from build123d import *

# Parameters (mm, degrees)
BOSS_EXTRUDE1_DEPTH = 17.5
SKETCH2_R           = 5
CUT_EXTRUDE1_DEPTH  = 36
SKETCH3_R           = 1.65
CUT_EXTRUDE2_DEPTH  = 27
FILLET1_R           = 0.7
SKETCH8_R           = 8
CUT_EXTRUDE5_DEPTH  = 1


with BuildPart() as part:
    # Sketch1 → Boss-Extrude1 (new body, symmetric)
    with BuildSketch(Plane(origin=(0, 0, 0), x_dir=(0, 0, -1), z_dir=(1, 0, 0))):
        Polygon((-20, 26), (-7, 26), (-7, 25), (7, 25), (7, 26), (20, 26), (20, 18), (18, 16), (18, 5), (9.980120734, 5), (5.980120734, 0), (-5.980120734, 0), (-9.980120734, 5), (-18, 5), (-18, 16), (-20, 18), align=None)
    extrude(amount=BOSS_EXTRUDE1_DEPTH, both=True)

    # Sketch2 → Cut-Extrude1 (cut, through all)
    with BuildSketch(Plane(origin=(17.5, 0, 0), x_dir=(0, 0, -1), z_dir=(1, 0, 0))):
        with Locations((0, 13)):
            Circle(SKETCH2_R)
    extrude(amount=-CUT_EXTRUDE1_DEPTH, mode=Mode.SUBTRACT)

    # Sketch3 → Cut-Extrude2 (cut, through all)
    with BuildSketch(Plane(origin=(0, 26, 0), x_dir=(1, 0, 0), z_dir=(0, 1, 0))):
        with Locations((-10.5, 14)):
            Circle(SKETCH3_R)
        with Locations((10.5, 14)):
            Circle(SKETCH3_R)
        with Locations((10.5, -14)):
            Circle(SKETCH3_R)
        with Locations((-10.5, -14)):
            Circle(SKETCH3_R)
    extrude(amount=-CUT_EXTRUDE2_DEPTH, mode=Mode.SUBTRACT)

    # Fillet1
    fillet1_edges = [part.edges().sort_by_distance(p)[0] for p in [
        (-12.15, 26, -14),
        (8.85, 26, -14),
        (8.85, 26, 14),
        (-12.15, 26, 14),
    ]]
    fillet(fillet1_edges, radius=FILLET1_R)

    # Sketch8 → Cut-Extrude5 (cut)
    with BuildSketch(Plane(origin=(17.5, 0, 0), x_dir=(0, 0, -1), z_dir=(1, 0, 0))):
        with Locations((0, 13)):
            Circle(SKETCH8_R)
    cut_extrude5 = extrude(amount=-CUT_EXTRUDE5_DEPTH, mode=Mode.SUBTRACT)

    # Mirror3: Cut-Extrude5 across plane
    add(cut_extrude5.mirror(Plane(origin=(0, 0, 0), x_dir=(0, 0, 1), z_dir=(1, 0, 0))), mode=Mode.SUBTRACT)


solid = part.part
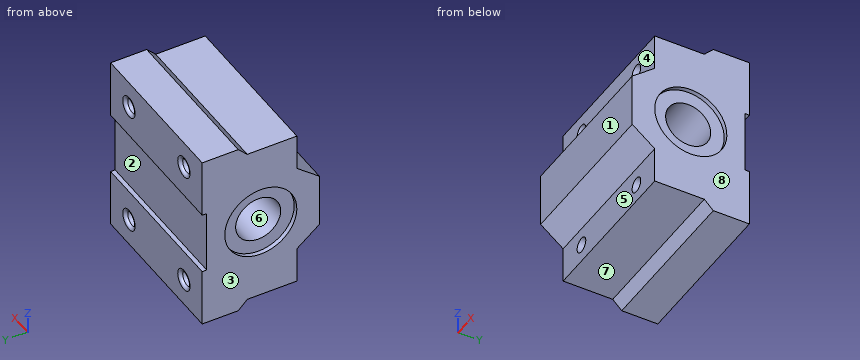
Source: CAD feature listing. Evaluate the final solid. Frame: model axes, mm. Face numbers are marked on the shaded views. A direction names the side the tool comes from. Give positions to 0.01 mm unless a question says otherwise; leave off trailing zeros. Write each loop counter-clockwise with the first axis right and the second up, starting at its lowest first coordinate (ties: lowest second). Pieces come first, ordered by that corner, then holes. Notation, with made-up numbers: M 57.25,59.25 L 76.25,59.25 A22 ccw 76.25,87.25 Z; hole C 56,-38 d1. An arc over 180 degrees is marked long. Answer as a JSON object with one key per item and string values.
Q1. Cut plane A-A, the plane y = 13. Return the cut outline in (x, z).
Geometry check:
{"outline": "M -17.5,-18 L 17.5,-18 L 17.5,-8 L 16.5,-8 L 16.5,-5 L -16.5,-5 L -16.5,-8 L -17.5,-8 Z; M -17.5,8 L -16.5,8 L -16.5,5 L 16.5,5 L 16.5,8 L 17.5,8 L 17.5,18 L -17.5,18 Z; hole C -10.5,-14 d3.3; hole C -10.5,14 d3.3; hole C 10.5,-14 d3.3; hole C 10.5,14 d3.3"}
Q2. Cut plane B-B, the plane x = 10.5. Count the separate pieces of the cut face and the enclosed holes in it, then the cut area to 3 significant figures.
Geometry check:
{"separate pieces": "3", "enclosed holes": "1", "area": "640 mm^2"}
Q3. Cut plane D-D, the plane y = 20.25. Return the cut outline in (x, z), then the cut area to 3 significant figures.
Geometry check:
{"outline": "M -17.5,-20 L 17.5,-20 L 17.5,-3.38 L 16.5,-3.38 L 16.5,3.38 L 17.5,3.38 L 17.5,20 L -17.5,20 L -17.5,3.38 L -16.5,3.38 L -16.5,-3.38 L -17.5,-3.38 Z; hole C -10.5,-14 d3.3; hole C -10.5,14 d3.3; hole C 10.5,-14 d3.3; hole C 10.5,14 d3.3", "area": "1,350 mm^2"}
Q4. Cut plane C-C, the plane z = 14. Return the cut outline in (x, y), then the cut area to 3 significant figures.
Geometry check:
{"outline": "M -17.5,5 L -12.15,5 L -12.15,25.3 A0.7 ccw -12.85,26 L -17.5,26 Z; M -8.85,5 L 8.85,5 L 8.85,25.3 A0.7 ccw 8.15,26 L -8.15,26 A0.7 ccw -8.85,25.3 Z; M 12.15,5 L 17.5,5 L 17.5,26 L 12.85,26 A0.7 ccw 12.15,25.3 Z", "area": "596 mm^2"}
Q5. Mould query, pull axis Z, two halves, no side actions, for the marked faces 6, 7 and 8. Classes: +Z half, -Z half, draft (parallel to the pull), parting line (faces both ways), or undercut.
Geometry check:
{"face 6": "undercut", "face 7": "-Z half", "face 8": "draft"}
Q6. Ray query, line 1 along Z through (x, y) = (-10.5, 18.25); line 2 along Z through (x, y) = (-10.5, 16); line 3 along Y through (x, z) = (-17.1, 0). Return the intervals inside material, ascending.
Geometry check:
{"line 1": "z = -20 to -15.65, -12.35 to 12.35, 15.65 to 20", "line 2": "z = -18 to -15.65, -12.35 to -4, 4 to 12.35, 15.65 to 18", "line 3": "y = 0 to 5, 21 to 25"}
Q7. Access query for the marked faces 1, 2, 3, 4 and 5. Directions: +Z, -Z, +X, -X, +Y, -Y. A direction counts if a zero-diameter tool reaches every point of the face in a straight line with its end or side. Return the directions, or none.
Geometry check:
{"face 1": "+Z, -Z, +X, -X, -Y", "face 2": "+X, -X, +Y", "face 3": "+Z, -Z, -X, +Y, -Y", "face 4": "+Z, +X, -X, -Y", "face 5": "-Z, +X, -X, -Y"}
Q8. Contact query for flat-ended pins moving along their axis: P1, Ø2.5, axis at x = 1, z = -15, coming from the -Y side; P2, Ø3, axis at x = -3.5, y = 9, coming from the +Z side; P3, Ø1.5, axis at x = 7, y = 3.5, coming from the -Z side; P4, Ø8, axis at y = 13, z = 0, coming from the +X side. Output: stop coordinate, or through.
Geometry check:
{"P1": "stops at y = 5", "P2": "stops at z = 18", "P3": "stops at z = -9.38", "P4": "passes through"}
